Work out the finished part from the listing and answer in its coordinate system (mm). Face numbers are marked on the shaded views. A direction names the side the tool comes from. Coordinates: 2 decimals unless noted, no trailing zeros. Order: outer loops, then holes, each group sorted by start corner. A loop starts at its lowest first (then second) coordinate and runs counter-clockwise, first axis right, second up.
1. The part is cut by section A-A, the plane z = 0. Give the vertices of the cut face in (x, y).
2. Find the intervals of material crossed by probe 1 along Y at (x, z) = (-3, -23); probe 2 along X at (y, z) = (3.75, 7); probe 3 along Y at (x, z) = (30, -9.5), in increasing order.
3. The part is cut by section D-D, the plane y = 9. Give the vertices of the cut face in (x, z).
4. The part is cut by section B-B, the plane x = 0. Give the vertices of the cut face in (y, z).
5. Flat-ended cylindrical pins translate along their axes: pin 1 Ø4.5 at (x, z) = (0, -32.5) entering from +Y; pin 2 Ø1 at (x, y) = (-3.5, 6) entering from -Z; pin 3 Ø1 at (y, z) = (5.5, 4) entering from +X; pin 4 Ø3 at (x, z) = (0, 32.5) entering from -Y. Find the tip coordinate at first contact, or state that the pin passes through.
6. A tool of negligible diameter and unlimited length cuts with its end or side. For the marked faces 1 and 2, from which of +Z, -Z, +X, -X, +Y, -Y can it reach the whole face along a straight path? Write none if from no direction.
7. The part is cut by section C-C, the plane z = -19.5. Give the vertices of the cut face in (x, y).
8. Determine the mould class of the marked faces 3, 4 and 5 for opening direction Z: +Z half, -Z half, draft (parallel to the pull), parting line (faces both ways), or undercut.
```python
from build123d import *

# Parameters (mm, degrees)
SKIZZE1_R                       = 37.5
SKIZZE1_R_2                     = 22
AUFSATZ_LINEAR_AUSTRAGEN1_DEPTH = 14
SCHNITT_LINEAR_START            = -6.5
SKIZZE2_R                       = 37.5
SKIZZE2_R_2                     = 27
SCHNITT_LINEAR_AUSTRAGEN1_DEPTH = 6.5
M4X0_7_GEWINDEBOHRUNG1_D        = 3.3
SKIZZE5_R                       = 26.5
SCHNITT_LINEAR_AUSTRAGEN2_DEPTH = 2


with BuildPart() as part:
    # Skizze1 → Aufsatz-Linear austragen1 (new body)
    with BuildSketch(Plane(origin=(0, 0, 0), x_dir=(1, 0, 0), z_dir=(0, 1, 0))):
        with Locations(Location((0, 0, 0), (0, 0, 270))):
            Circle(SKIZZE1_R)
        with Locations(Location((0, 0, 0), (0, 0, 270))):
            Circle(SKIZZE1_R_2, mode=Mode.SUBTRACT)
    extrude(amount=AUFSATZ_LINEAR_AUSTRAGEN1_DEPTH)

    # Skizze2 → Schnitt-Linear austragen1 (cut)
    with BuildSketch(Plane(origin=(0, 14, 0), x_dir=(1, 0, 0), z_dir=(0, 1, 0)).offset(SCHNITT_LINEAR_START)):
        with Locations(Location((0, 0, 0), (0, 0, 270))):
            Circle(SKIZZE2_R)
        with Locations(Location((0, 0, 0), (0, 0, 270))):
            Circle(SKIZZE2_R_2, mode=Mode.SUBTRACT)
    extrude(amount=SCHNITT_LINEAR_AUSTRAGEN1_DEPTH, mode=Mode.SUBTRACT)

    # M4x0.7 Gewindebohrung1 (through all)
    with Locations(Plane(origin=(0, 7.5, 0), x_dir=(1, 0, 0), z_dir=(0, 1, 0))):
        with Locations((-32.5, 0), (0, 32.5), (0, -32.5), (32.5, 0)):
            Hole(M4X0_7_GEWINDEBOHRUNG1_D / 2)

    # Skizze5 → Schnitt-Linear austragen2 (cut)
    with BuildSketch(Plane.XZ):
        with Locations(Location((0, 0, 0), (0, 0, 270))):
            Circle(SKIZZE5_R)
    extrude(amount=-SCHNITT_LINEAR_AUSTRAGEN2_DEPTH, mode=Mode.SUBTRACT)


solid = part.part
```
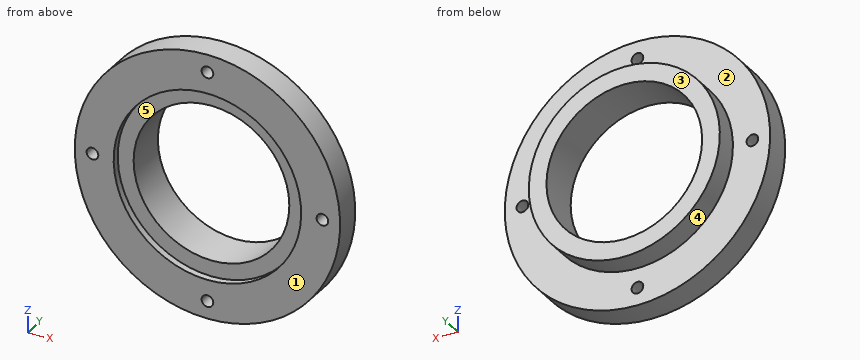
Geometry says:
1. outline: (-37.5, 0) - (-34.15, 0) - (-34.15, 7.5) - (-37.5, 7.5) - close; (-30.85, 0) - (-26.5, 0) - (-26.5, 2) - (-22, 2) - (-22, 14) - (-27, 14) - (-27, 7.5) - (-30.85, 7.5) - close; (22, 2) - (26.5, 2) - (26.5, 0) - (30.85, 0) - (30.85, 7.5) - (27, 7.5) - (27, 14) - (22, 14) - close; (34.15, 0) - (37.5, 0) - (37.5, 7.5) - (34.15, 7.5) - close
2. probe 1: y = 2 to 14
2. probe 2: x = -36.84 to -20.86, 20.86 to 36.84
2. probe 3: y = 0 to 7.5
3. outline: circle Ø54 at (0, 0); hole circle Ø44 at (0, 0)
4. outline: (0, -37.5) - (7.5, -37.5) - (7.5, -34.15) - (0, -34.15) - close; (0, -30.85) - (7.5, -30.85) - (7.5, -27) - (14, -27) - (14, -22) - (2, -22) - (2, -26.5) - (0, -26.5) - close; (0, 26.5) - (2, 26.5) - (2, 22) - (14, 22) - (14, 27) - (7.5, 27) - (7.5, 30.85) - (0, 30.85) - close; (0, 34.15) - (7.5, 34.15) - (7.5, 37.5) - (0, 37.5) - close
5. pin 1: stops at y = 7.5
5. pin 2: stops at z = -37.38
5. pin 3: stops at x = 37.34
5. pin 4: passes through
6. face 1: +Z, -Z, +X, -X, -Y
6. face 2: +Y
7. outline: (-32.03, 0) - (-17.94, 0) - (-17.94, 2) - (-10.19, 2) - (-10.19, 14) - (-18.67, 14) - (-18.67, 7.5) - (-32.03, 7.5) - close; (10.19, 2) - (17.94, 2) - (17.94, 0) - (32.03, 0) - (32.03, 7.5) - (18.67, 7.5) - (18.67, 14) - (10.19, 14) - close
8. face 3: draft
8. face 4: parting line
8. face 5: undercut
